Autodesk Inventor part; units mm, degrees
ref_plane "YZ Plane" through (0, 0, 0) normal (1, 0, 0) x (0, 1, 0)
ref_plane "XZ Plane" through (0, 0, 0) normal (0, 1, 0) x (-1, 0, 0)
ref_plane "XY Plane" through (0, 0, 0) normal (0, 0, 1) x (1, 0, 0)
ref_plane "Arbeitsebene1" through (0, 0, 0) normal (0, 0, 1) x (1, 0, 0)
sketch "Skizze1" plane through (0, 0, 0) normal (0, 0, 1) x (1, 0, 0)
  circle A0 centre (-34, -41.2095) radius 2.25
  line L0 (-29.75, -46.3143) -> (-39, -46.3143)
  line L1 (-29.75, -28.7171) -> (-29.75, -46.3143)
  line L2 (-31, -28.7171) -> (-29.75, -28.7171)
  arc A1 (-31, -28.7171) -> (-39, -36.7171) centre (-31, -36.7171) ccw
  line L3 (-39, -46.3143) -> (-39, -36.7171)
  line L4 (22, 46.3143) -> (22, 27.3143)
  line L5 (14, 46.3143) -> (22, 46.3143)
  line L6 (14, 27.3143) -> (14, 46.3143)
  line L7 (22, 27.3143) -> (14, 27.3143)
  circle A2 centre (18, 30.3143) radius 2.25
  circle A3 centre (18, 41.3143) radius 3.2
  line L8 (39, -36.6857) -> (39, -43.7095)
  arc A4 (39, -36.6857) -> (31, -28.6857) centre (31, -36.6857) ccw
  line L9 (30, -28.6857) -> (31, -28.6857)
  arc A5 (22, -20.6857) -> (30, -28.6857) centre (30, -20.6857) ccw
  line L10 (22, -18.1808) -> (22, -20.6857)
  line L11 (20, -18.1808) -> (22, -18.1808)
  line L12 (20, -43.7095) -> (20, -18.1808)
  line L13 (39, -43.7095) -> (20, -43.7095)
  circle A6 centre (34, -39.4595) radius 2.25
  circle A7 centre (34, -58.6857) radius 4.25 construction
  circle A8 centre (-34, -58.6857) radius 4.25 construction
  circle A9 centre (18, 41.3143) radius 3.2 construction
  circle A10 centre (34, -39.4595) radius 2.25 construction
  circle A11 centre (-34, -41.2095) radius 2.25 construction
  circle A12 centre (18, 30.3143) radius 2.25 construction
  circle A13 centre (18, -14.7167) radius 2 construction
  circle A14 centre (18, 8.8143) radius 2 construction
  circle A15 centre (3.8024, -65.6857) radius 18.5 construction
  circle A16 centre (3, -8.6688) radius 3.05 construction
  arc A17 (-31, -28.7171) -> (-39, -36.7171) centre (-31, -36.7171) ccw construction
  line L14 (-11, -28.7171) -> (-31, -28.7171) construction
  arc A18 (-11, -28.7171) -> (-3, -20.7171) centre (-11, -20.7171) ccw construction
  line L15 (-3, 17.3143) -> (-3, -20.7171) construction
  arc A19 (5, 25.3143) -> (-3, 17.3143) centre (5, 17.3143) ccw construction
  line L16 (14, 25.3143) -> (5, 25.3143) construction
  line L17 (14, 46.3143) -> (14, 25.3143) construction
  line L18 (22, 46.3143) -> (14, 46.3143) construction
  line L19 (22, -20.6857) -> (22, 46.3143) construction
  arc A20 (22, -20.6857) -> (30, -28.6857) centre (30, -20.6857) ccw construction
  line L20 (31, -28.6857) -> (30, -28.6857) construction
  arc A21 (39, -36.6857) -> (31, -28.6857) centre (31, -36.6857) ccw construction
  line L21 (39, -79.0756) -> (39, -36.6857) construction
  arc A22 (31, -87.0756) -> (39, -79.0756) centre (31, -79.0756) ccw construction
  line L22 (-31, -87.0756) -> (31, -87.0756) construction
  arc A23 (-39, -79.0756) -> (-31, -87.0756) centre (-31, -79.0756) ccw construction
  line L23 (-39, -36.7171) -> (-39, -79.0756) construction
  circle A24 centre (3, 16.3312) radius 4
  circle A25 centre (3, -33.6688) radius 4
  circle A26 centre (3, 16.3312) radius 7.6
  circle A27 centre (3, 16.3312) radius 4
  circle A28 centre (3, 16.3312) radius 6
  circle A29 centre (3, 16.3312) radius 6
  line L24 (-39, -46.3143) -> (39, -46.3143)
  line L25 (39, -46.3143) -> (39, -43.7095)
  line L26 (-29.75, -28.7171) -> (-3, -28.7171)
  line L27 (-3, -28.7171) -> (-3, 46.3143)
  line L28 (-3, 46.3143) -> (22, 46.3143)
  line L29 (22, 46.3143) -> (22, -18.1808)
  line L30 (22, 46.3143) -> (57, 46.3143)
  line L31 (57, 46.3143) -> (57, -37.6857)
  line L32 (57, -37.6857) -> (22, -37.6857)
  line L33 (22, -37.6857) -> (22, 46.3143)
  line L34 (39, -46.3143) -> (57, -46.3143)
  line L35 (57, -46.3143) -> (57, -37.6857)
  line L36 (57, -37.6857) -> (39, -37.6857)
  line L37 (39, -37.6857) -> (39, -46.3143)
  point P0 (0, 0)
  dimension "d10" = 84
  dimension "d11" = 60
extrude "Extrusion1" add sketch "Skizze1" along normal blind 3 contours L0 L3 A1 L2 L1 | L1 L26 L27 A26 L28 L6 L7 L29 L11 L12 L13 L25 L24 | L25 L8 L32 L35 L34 | L13 L12 L11 L10 L33 L32 A6 L8 | A28 | L27 A26 | L32 A6 L33 A5 L9 A4 L8 | L8 A4 L9 A5 L10 L29 L4 L30 L31 L32 | L32 A6 | L4 L7 L6 L5 | A24 | A25 picked at (9.931, 15.2305) picked at (34.3207, -37.599)
sketch "Skizze2" plane through (0, 0, 0) normal (0, 0, -1) x (-1, 0, 0)
  circle A0 centre (-3, 16.3312) radius 4
  circle A1 centre (-3, -33.6688) radius 4
  circle A2 centre (-3, 16.3312) radius 4.3
  circle A3 centre (-3, -33.6688) radius 4.3
  circle A4 centre (-3, 16.3312) radius 6
  circle A5 centre (-3, -33.6688) radius 6
  point P0 (0, 0)
  dimension "d2" = 0.3
  dimension "d3" = 0.3
  dimension "d4" = 1.7
  dimension "d5" = 1.7
extrude "Extrusion2" add sketch "Skizze2" along normal blind 3 contours A4 | A5
sketch "Skizze3" plane through (0, 0, 3) normal (0, 0, 1) x (1, 0, 0)
  circle A0 centre (18, 41.3143) radius 3.2
  circle A1 centre (18, 30.3143) radius 2.25
  arc A2 (32.6157, -37.6857) -> (35.3843, -37.6857) centre (34, -39.4595) ccw
  circle A3 centre (-34, -41.2095) radius 2.25
  point P0 (0, 0)
hole "Bohrung1" at (18, 41.3143, 3) at (18, 30.3143, 3) at (34, -39.4595, 3) at (-34, -41.2095, 3) direction (0, 0, -1) diameter 4 end through all countersink diameter 10 countersink angle 90
properties part number "11_Smartphone_Platform"
Geometry check sheet. Reference: the model listing, model coordinates, mm. A direction names the side the tool comes from. Coordinates: 2 decimals unless noted, no trailing zeros. Write each loop counter-clockwise with the first axis right and the second up, starting at its lowest first coordinate (ties: lowest second). Pieces come first, ordered by that corner, then holes. Notation, with made-up numbers: M 79.5,82.25 L 97.5,82.25 A14 ccw 97.5,93.25 Z; hole C 74.25,-28 d7. An arc over 180 degrees is marked long. Use one line per item in the form item = value. Start each with the question number.
1) Go/stop test with flat-tipped pins: pin 1 Ø1.5 at (y, z) = (31.5, 2) entering from -X; pin 2 Ø4.5 at (x, y) = (3.5, -33.5) entering from -Z; pin 3 Ø6 at (x, y) = (-34, -41.21) entering from +Z; pin 4 Ø3.5 at (x, y) = (18, 30.31) entering from +Z. Record where each tip stops, or that it passes through.
2) Set-up check for faces 1 (the cylindrical face through (3.56, -37.932, -1.479)), 2 (the flat face through (57, -1, 1)): record each of +Z, -Z, +X, -X, +Y, -Y from which the full face is reachable in a straight line by a thin tool's end or side.
3) Section check D-D on y = -32.5. Enter the section's corners in (x, z).
4) Section check B-B on x = 3. Enter the section's corners in (y, z).
5) Release check for a two-part mould opening along Y. For faces 3 (the flat face through (3, -34, 0)), 4 (the conical face through (16.731, 38.254, 1.313)), 5 (the flat face through (-39, -42, 1)), 6 (the cylindrical face through (-36.719, -31.123, 1.479)) record: pulls with the +Y half, pulls with the -Y half, needs draft (parallel to the pull), parting line crosses it, or undercut.
6) Section check A-A on x = -34. Enter the section's corners in (y, z).
7) Section check C-C on y = -9.5. Enter the section's corners in (x, z).
8) Thickness scan on probe 1 along Y at (x, z) = (18, 0.1); probe 2 along X at (y, z) = (-40, 1); probe 3 along Y at (x, z) = (4, -0.15). Record the ranges inside material, lowest first. Write a range as from..to.
Responses:
q1.pin_1 = -3
q1.pin_2 = 0
q1.pin_3 = 1
q1.pin_4 = through
q2.face_1 = -Z
q2.face_2 = +Z, -Z, +X, +Y, -Y
q3.outline = M -37.8,0 L -2.89,0 L -2.89,-3 L -1.14,-3 L -1.14,0 L 7.14,0 L 7.14,-3 L 8.89,-3 L 8.89,0 L 57,0 L 57,3 L -37.8,3 Z
q4.outline = M -46.31,0 L -39.67,0 L -39.67,-3 L -37.97,-3 L -37.97,0 L -29.37,0 L -29.37,-3 L -27.67,-3 L -27.67,0 L 10.33,0 L 10.33,-3 L 12.03,-3 L 12.03,0 L 20.63,0 L 20.63,-3 L 22.33,-3 L 22.33,0 L 46.31,0 L 46.31,3 L -46.31,3 Z
q5.face_3 = undercut
q5.face_4 = undercut
q5.face_5 = needs draft
q5.face_6 = pulls with the +Y half
q6.outline = M -46.31,0 L -43.46,0 L -43.46,0.25 L -46.21,3 L -46.31,3 Z; M -38.96,0 L -29.3,0 L -29.3,3 L -36.21,3 L -38.96,0.25 Z
q7.outline = M -3,0 L 57,0 L 57,3 L -3,3 Z
q8.probe_1 = -46.31..28.06, 32.56..38.11, 44.51..46.31
q8.probe_2 = -39..-36.75, -31.25..31.05, 36.95..57
q8.probe_3 = -39.58..-37.85, -29.49..-27.75, 10.42..12.15, 20.51..22.25
